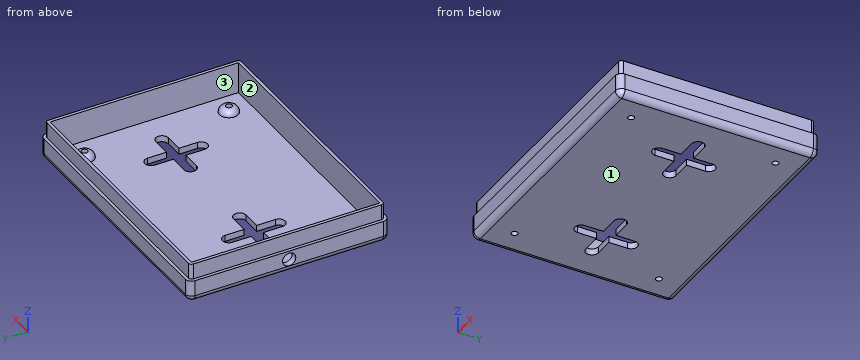
from build123d import *

# Parameters (mm, degrees)
BOX_W           = 80
BOX_H           = 60
BOX_DEPTH       = 10
THICKNESS_T     = 2
POCKET_DEPTH    = 5
SKETCH006_R     = 1
POCKET001_DEPTH = 12.001
POCKET002_DEPTH = 12.001
SKETCH011_R     = 2.1
POCKET003_DEPTH = 2


with BuildPart() as standoff:
    # Sketch010 → Revolution (revolve)
    with BuildSketch(Plane.XZ):
        with BuildLine():
            ThreePointArc((-1, 2), (-2.414214, 1.414214), (-3, 0))
            Line((-3, 0), (0, 0))
            Line((0, 2), (0, 0))
            Line((-1, 2), (0, 2))
        make_face()
    revolve(axis=Axis((0, 0, 0), (0, 0, 1)))


with BuildPart() as standofftopleft:
    # Clone004 base: copy of StandOff
    add(standoff.part)


with BuildPart() as standofftopleft_1:
    # Clone004 placement: moved
    add(standofftopleft.part.moved(Location((7, 53, 0))))


with BuildPart() as standofftopright:
    # Clone005 base: copy of StandOff
    add(standoff.part)


with BuildPart() as standofftopright_1:
    # Clone005 placement: moved
    add(standofftopright.part.moved(Location((73, 53, 0))))


with BuildPart() as standoffbottomright:
    # Clone006 base: copy of StandOff
    add(standoff.part)


with BuildPart() as standoffbottomright_1:
    # Clone006 placement: moved
    add(standoffbottomright.part.moved(Location((73, 7, 0))))


with BuildPart() as standoffbottomleft:
    # Clone007 base: copy of StandOff
    add(standoff.part)


with BuildPart() as standoffbottomleft_1:
    # Clone007 placement: moved
    add(standoffbottomleft.part.moved(Location((7, 7, 0))))


with BuildPart() as obj1:
    # Box → Box (new body)
    with BuildSketch(Plane.XY):
        with Locations((40, 30)):
            Rectangle(BOX_W, BOX_H)
    extrude(amount=BOX_DEPTH)

    # Thickness
    thickness_openings = [obj1.faces().sort_by_distance(p)[0] for p in [
        (40, 30, 10),
    ]]
    offset(amount=THICKNESS_T, openings=thickness_openings)

    # Sketch004 → Pocket (cut)
    with BuildSketch(Plane.XY.offset(10)):
        with BuildLine():
            Line((0, 62), (80, 62))
            ThreePointArc((82, 60), (81.414214, 61.414214), (80, 62))
            Line((82, 60), (82, 0))
            ThreePointArc((80, -2), (81.414214, -1.414214), (82, 0))
            Line((80, -2), (0, -2))
            ThreePointArc((-2, 0), (-1.414214, -1.414214), (0, -2))
            Line((-2, 0), (-2, 60))
            ThreePointArc((0, 62), (-1.414214, 61.414214), (-2, 60))
        make_face()
        with BuildLine():
            Line((0, 61), (80, 61))
            ThreePointArc((81, 60), (80.707107, 60.707107), (80, 61))
            Line((81, 60), (81, 0))
            ThreePointArc((80, -1), (80.707107, -0.707107), (81, 0))
            Line((80, -1), (0, -1))
            ThreePointArc((-1, 0), (-0.707107, -0.707107), (0, -1))
            Line((-1, 0), (-1, 60))
            ThreePointArc((0, 61), (-0.707107, 60.707107), (-1, 60))
        make_face(mode=Mode.SUBTRACT)
    extrude(amount=-POCKET_DEPTH, mode=Mode.SUBTRACT)

    # Fusion002: union StandOffTopLeft, StandOffTopRight, StandOffBottomRight, StandOffBottomLeft
    add(standofftopleft_1.part)
    add(standofftopright_1.part)
    add(standoffbottomright_1.part)
    add(standoffbottomleft_1.part)

    # Sketch006 → Pocket001 (cut, through all)
    with BuildSketch(Plane(origin=(0, 0, -2), x_dir=(1, 0, 0), z_dir=(0, 0, -1))):
        with Locations((7, -7)):
            Circle(SKETCH006_R)
        with Locations((7, -53)):
            Circle(SKETCH006_R)
        with Locations((73, -53)):
            Circle(SKETCH006_R)
        with Locations((73, -7)):
            Circle(SKETCH006_R)
    extrude(amount=-POCKET001_DEPTH, mode=Mode.SUBTRACT)

    # Sketch009 → Pocket002 (cut, through all)
    with BuildSketch(Plane(origin=(0, 0, -2), x_dir=(1, 0, 0), z_dir=(0, 0, -1))):
        with BuildLine():
            Line((10, -28), (16, -28))
            Line((16, -28), (16, -22))
            ThreePointArc((20, -22), (18, -20), (16, -22))
            Line((20, -22), (20, -28))
            Line((20, -28), (26, -28))
            ThreePointArc((26, -32), (28, -30), (26, -28))
            Line((26, -32), (20, -32))
            Line((20, -32), (20, -38))
            ThreePointArc((16, -38), (18, -40), (20, -38))
            Line((16, -38), (16, -32))
            Line((16, -32), (10, -32))
            ThreePointArc((10, -28), (8, -30), (10, -32))
        make_face()
        with BuildLine():
            ThreePointArc((54, -28), (52, -30), (54, -32))
            Line((54, -32), (60, -32))
            Line((60, -32), (60, -38))
            ThreePointArc((60, -38), (62, -40), (64, -38))
            Line((64, -38), (64, -32))
            Line((64, -32), (70, -32))
            ThreePointArc((70, -32), (72, -30), (70, -28))
            Line((70, -28), (64, -28))
            Line((64, -22), (64, -28))
            ThreePointArc((64, -22), (62, -20), (60, -22))
            Line((60, -28), (60, -22))
            Line((54, -28), (60, -28))
        make_face()
    extrude(amount=-POCKET002_DEPTH, mode=Mode.SUBTRACT)

    # Sketch011 → Pocket003 (cut)
    with BuildSketch(Plane(origin=(-2, 0, 0), x_dir=(0, -1, 0), z_dir=(-1, 0, 0))):
        with Locations((-30, 2.2)):
            Circle(SKETCH011_R)
    extrude(amount=-POCKET003_DEPTH, mode=Mode.SUBTRACT)


solid = obj1.part
The model under review builds one solid part; all positions refer to its coordinate system, in mm. Face numbers are marked on the shaded views. Round coordinates to 2 decimals unless told otherwise and drop trailing zeros. Loops run counter-clockwise (first coordinate to the right, second up) from the corner with the lowest first, then second, coordinate; pieces in that order, holes last. Notation, with made-up numbers: M -21.75,70.25 L 21.25,70.25 A21 ccw 21.25,94.25 Z; hole C -20,43.5 d2. An arc over 180 degrees is marked long. Answer as a JSON object with one key per item and string values.
Item 1: For line 1 along Y through (x, z) = (7, 0.05); line 2 along Y through (x, z) = (44, 2); line 3 along Y through (x, z) = (7, 0.7), list the stretches that pass through material, from the lowest coordinate up.
Check sheet entries:
{"line 1": "-2 to 0, 4 to 6, 8 to 10, 50 to 52, 54 to 56, 60 to 62", "line 2": "-2 to 0, 60 to 62", "line 3": "-2 to 0, 4.13 to 6, 8 to 9.87, 50.13 to 52, 54 to 55.87, 60 to 62"}
Item 2: We need section D-D, the plane z = 7.5. State the section outline as (x, y) points, and give its area (3 significant figures).
Check sheet entries:
{"outline": "M -1,0 A1 ccw 0,-1 L 80,-1 A1 ccw 81,0 L 81,60 A1 ccw 80,61 L 0,61 A1 ccw -1,60 Z; hole M 0,0 L 80,0 L 80,60 L 0,60 Z", "area": "283 mm2"}
Item 3: We need section A-A, the plane y = 30. State the section outline as (x, z) points.
Check sheet entries:
{"outline": "M -2,0 A2 ccw 0,-2 L 8,-2 L 8,0 L 0,0 L 0,0.1 L -2,0.1 Z; M -2,4.3 L 0,4.3 L 0,10 L -1,10 L -1,5 L -2,5 Z; M 28,-2 L 52,-2 L 52,0 L 28,0 Z; M 72,-2 L 80,-2 A2 ccw 82,0 L 82,5 L 81,5 L 81,10 L 80,10 L 80,0 L 72,0 Z"}
Item 4: Clearance check with flat-ended pins moving along their axes: P1, Ø1.5, axis at y = 18, z = 6.5, coming from the +X side; P2, Ø1.8, axis at x = 73, y = 7, coming from the +Z side; P3, Ø2, axis at x = 34.5, y = 7.5, coming from the +Z side; P4, Ø5, axis at x = 20, z = 5.5, coming from the +Y side. State where each tip first meets the part, or that it passes through.
Check sheet entries:
{"P1": "x = 81", "P2": "through", "P3": "z = 0", "P4": "y = 62"}
Item 5: We need section B-B, the plane x = 41. State the section outline as (y, z) points, and give its area (3 significant figures).
Check sheet entries:
{"outline": "M -2,0 A2 ccw 0,-2 L 60,-2 A2 ccw 62,0 L 62,5 L 61,5 L 61,10 L 60,10 L 60,0 L 0,0 L 0,10 L -1,10 L -1,5 L -2,5 Z", "area": "156 mm2"}
Item 6: The part is to be moulded in two halves that separate along Y. For the marked faces 1, 2 and 3, say which applies: +Y half, -Y half, draft (parallel to the pull), parting line (faces both ways), or undercut.
Check sheet entries:
{"face 1": "draft", "face 2": "undercut", "face 3": "undercut"}
Item 7: We need section C-C, the plane y = 23. State the section outline as (x, z) points, and give its area (3 significant figures).
Check sheet entries:
{"outline": "M -2,0 A2 ccw 0,-2 L 16,-2 L 16,0 L 0,0 L 0,10 L -1,10 L -1,5 L -2,5 Z; M 20,-2 L 60,-2 L 60,0 L 20,0 Z; M 64,-2 L 80,-2 A2 ccw 82,0 L 82,5 L 81,5 L 81,10 L 80,10 L 80,0 L 64,0 Z", "area": "180 mm2"}
